The model under review builds one solid part; all positions refer to its coordinate system, in mm. A direction names the side the tool comes from. Coordinates: 2 decimals unless noted, no trailing zeros. Loops run counter-clockwise (first coordinate to the right, second up) from the corner with the lowest first, then second, coordinate; pieces in that order, holes last. Notation, with made-up numbers: M 32,26 L 78,26 A11 ccw 78,41 Z; hole C -2,-15 d6. An arc over 180 degrees is marked long. Write item = value, one per line. Start each with the question number.
Q1. Wall thickness on probe 1 along X at (y, z) = (0, 4.25); probe 2 along X at (y, z) = (0.5, -5); probe 3 along X at (y, z) = (-1.25, -4): over which ranges is each line inside the solid? List them lowest first.
Q2. We need section C-C on x = 1. Give the boundary of the cut face in (y, z).
Q3. Clearance check with flat-ended pins moving along their axes: pin 1 Ø1 at (y, z) = (-2.5, -3.5) entering from -X; pin 2 Ø1.1 at (x, y) = (2, -2) entering from -Z; pin 3 Ø2 at (y, z) = (-0.5, 3) entering from +X. State where each tip first meets the part, or that it passes through.
Q4. We need section A-A on z = 1.5. Give the boundary of the cut face in (x, y), and give its area (3 significant figures).
Q5. We need section D-D on y = 2.75. Give the boundary of the cut face in (x, z), and give its area (3 significant figures).
Q6. For faces 1 (the face through (2.14, -1.65, 2.83)), 2 (the face through (-5.46, -1.67, 2.83)), 3 (the face through (0, 0, 0)), 4 (the face through (2.16, 1.67, 2.83)), list the 3-axis set-ups (+Z, -Z, +X, -X, +Y, -Y) from which the entire face can be reached by the end or side of a thin tool; tool diameter is ignored.
Q7. Mouldability with a two-part tool opening along Z and no side actions: class faces 5 (the face through (-3.87, 0.02, -1.83)), 6 (the face through (-5.48, 1.65, 2.83)), 7 (the face through (4, 0, 5.81)) as released by +Z, released by -Z, zero draft, split by the parting line, or undercut.
Q8. We need section B-B on y = -3. Give the boundary of the cut face in (x, z), and give its area (3 significant figures).
Autodesk Fusion 360 part; units mm, degrees
sketch "Baseplate" plane through (0, 0, 0) normal (0, 0, 1) x (1, 0, 0)
  line L0 (-7.239, 3.7465) -> (7.239, 3.7465)
  line L1 (7.239, 3.7465) -> (7.239, -3.7465)
  line L2 (7.239, -3.7465) -> (-7.239, -3.7465)
  line L3 (-7.239, -3.7465) -> (-7.239, 3.7465)
  line L4 (-7.239, 3.7465) -> (7.239, -3.7465) construction
  line L5 (7.239, 3.7465) -> (-7.239, -3.7465) construction
  dimension "d1" = 14.478
  dimension "d2" = 7.493
extrude "Extrude1" add sketch "Baseplate" against normal blind 2.159
sketch "UpperJoint" plane through (0, 0, 0) normal (0, 0, 1) x (-1, 0, 0)
  line L0 (7.239, 3.7465) -> (-7.239, 3.7465)
  line L1 (-7.239, 3.7465) -> (-7.239, -3.7465)
  line L2 (-7.239, -3.7465) -> (7.239, -3.7465)
  line L3 (7.239, -3.7465) -> (7.239, 3.7465)
  circle A0 centre (-3.81, 0) radius 2.54 construction
  line L4 (-4.782, -2.3467) -> (-2.838, -2.3467)
  line L5 (-2.838, -2.3467) -> (-1.4633, -0.972)
  line L6 (-1.4633, -0.972) -> (-1.4633, 0.972)
  line L7 (-1.4633, 0.972) -> (-2.838, 2.3467)
  line L8 (-2.838, 2.3467) -> (-4.782, 2.3467)
  line L9 (-4.782, 2.3467) -> (-6.1567, 0.972)
  line L10 (-6.1567, 0.972) -> (-6.1567, -0.972)
  line L11 (-6.1567, -0.972) -> (-4.782, -2.3467)
  line L12 (0, -2.5) -> (0, -20)
  line L13 (2.838, 2.3467) -> (4.782, 2.3467)
  line L14 (4.782, 2.3467) -> (6.1567, 0.972)
  line L15 (6.1567, 0.972) -> (6.1567, -0.972)
  line L16 (6.1567, -0.972) -> (4.782, -2.3467)
  line L17 (4.782, -2.3467) -> (2.838, -2.3467)
  line L18 (2.838, -2.3467) -> (1.4633, -0.972)
  line L19 (1.4633, -0.972) -> (1.4633, 0.972)
  line L20 (1.4633, 0.972) -> (2.838, 2.3467)
  point P0 (-3.81, 0)
  dimension "d5" = 5.08
  dimension "d7" = 3.81
extrude "Extrude2" add sketch "UpperJoint" along normal blind 5.81 contours L4 L5 L6 L7 L8 L9 L10 L11 | L13 L14 L15 L16 L17 L18 L19 L20
sketch "LegJoints" plane through (0, 0, 0) normal (1, 0, 0) x (0, 1, 0)
  circle A0 centre (0, -5.334) radius 3.5052
  dimension "d10" = 7.0104
  dimension "d11" = 5.334
extrude "Extrude3" cut sketch "LegJoints" along normal mid plane 20
extrude "Extrude4" add sketch "LegJoints" along normal mid plane 1.3
sketch "LegJoints2" plane through (-0.65, 0, 0) normal (-1, 0, 0) x (0, -1, 0)
  arc A0 (-1.4852, -2.159) -> (1.4852, -2.159) centre (0, -5.334) ccw
  arc A1 (1.4852, -2.159) -> (-1.4852, -2.159) centre (0, -5.334) ccw
  circle A2 centre (0, -5.334) radius 0.8255
  dimension "d16" = 1.651
extrude "Extrude5" add sketch "LegJoints2" along normal blind 5.08 contours A2
mirror "Mirror1" about plane through (0, 0, 0) normal (1, 0, 0) of "Extrude5"
fillet "Fillet1" radius 0.0635 2 edges at (5.73, 0.7696, -5.6325) (-5.73, 0.7696, -5.6325) 6 faces at (4.5922, 0.324, 5.81) (-3.0278, -0.324, 5.81) (2.413, 3.7465, -1.4393) (-7.239, 0, -0.6096) (7.239, 0, -0.6096) (-2.413, -3.7465, -1.4393)
Returned:
q1.probe_1 = -6.16 to -1.46, 1.46 to 6.16
q1.probe_2 = -5.73 to 5.73
q1.probe_3 = -0.65 to 0.65
q2.outline = M -3.75,-2.1 A0.06 ccw -3.68,-2.16 L -1.49,-2.16 A3.51 cw 1.49,-2.16 L 3.68,-2.16 A0.06 ccw 3.75,-2.1 L 3.75,-0.06 A0.06 ccw 3.68,0 L -3.68,0 A0.06 ccw -3.75,-0.06 Z; C 0,-5.33 d1.65
q3.pin_1 = -0.65
q3.pin_2 = -2.16
q3.pin_3 = 6.16
q4.outline = M -6.16,-0.97 L -4.78,-2.35 L -2.84,-2.35 L -1.46,-0.97 L -1.46,0.97 L -2.84,2.35 L -4.78,2.35 L -6.16,0.97 Z; M 1.46,-0.97 L 2.84,-2.35 L 4.78,-2.35 L 6.16,-0.97 L 6.16,0.97 L 4.78,2.35 L 2.84,2.35 L 1.46,0.97 Z
q4.area = 36.5 mm^2
q5.outline = M -7.24,-2.1 A0.06 ccw -7.18,-2.16 L 7.18,-2.16 A0.06 ccw 7.24,-2.1 L 7.24,-0.06 A0.06 ccw 7.18,0 L -7.18,0 A0.06 ccw -7.24,-0.06 Z; M -0.65,-7.51 L 0.65,-7.51 L 0.65,-3.16 L -0.65,-3.16 Z
q5.area = 36.9 mm^2
q6.face_1 = +Z, -Y
q6.face_2 = +Z, -X, -Y
q6.face_3 = +Z
q6.face_4 = +Z, +Y
q7.face_5 = undercut
q7.face_6 = zero draft
q7.face_7 = released by +Z
q8.outline = M -7.24,-2.1 A0.06 ccw -7.18,-2.16 L 7.18,-2.16 A0.06 ccw 7.24,-2.1 L 7.24,-0.06 A0.06 ccw 7.18,0 L -7.18,0 A0.06 ccw -7.24,-0.06 Z; M -0.65,-7.15 L 0.65,-7.15 L 0.65,-3.52 L -0.65,-3.52 Z
q8.area = 36.0 mm^2
